```python
from build123d import *

# Parameters (mm, degrees)
SKETCH1_W           = 57
SKETCH1_H           = 100
BOSS_EXTRUDE1_DEPTH = 80
SKETCH3_W           = 75
SKETCH3_H           = 90
CUT_EXTRUDE1_DEPTH  = 52
SKETCH4_R           = 4.025
CUT_EXTRUDE2_DEPTH  = 114.213294272
BOSS_EXTRUDE2_DEPTH = 30
CUT_EXTRUDE5_REACH  = 112.223
SKETCH8_W           = 85
SKETCH8_H           = 40
SKETCH5_R           = 5
SKETCH5_R_2         = 1.5
CUT_EXTRUDE3_DEPTH  = 141.791512528
SKETCH9_R           = 11
SKETCH9_R_2         = 3
CUT_EXTRUDE6_DEPTH  = 47.5
FILLET1_R           = 1
FILLET2_R           = 5


with BuildPart() as part:
    # Sketch1 → Boss-Extrude1 (new body)
    with BuildSketch(Plane(origin=(0, 0, 0), x_dir=(1, 0, 0), z_dir=(0, 1, 0))):
        Rectangle(SKETCH1_W, SKETCH1_H)
    extrude(amount=BOSS_EXTRUDE1_DEPTH)

    # Sketch3 → Cut-Extrude1 (cut)
    with BuildSketch(Plane(origin=(28.5, 40, 0), x_dir=(0, 1, 0), z_dir=(-1, 0, 0))):
        with Locations((2.5, 0)):
            Rectangle(SKETCH3_W, SKETCH3_H)
    extrude(amount=CUT_EXTRUDE1_DEPTH, mode=Mode.SUBTRACT)

    # Sketch4 → Cut-Extrude2 (cut, through all)
    with BuildSketch(Plane(origin=(-40, 5, 0), x_dir=(-1, 0, 0), z_dir=(0, -1, 0))):
        with Locations(Location((-40, 0, 0), (0, 0, 90))):
            Circle(SKETCH4_R)
    extrude(amount=CUT_EXTRUDE2_DEPTH, mode=Mode.SUBTRACT)

    # Sketch7 → Boss-Extrude2 (add)
    with BuildSketch(Plane.ZY.offset(28.5)):
        Polygon((-50, 80), (-42.5, 80), (-42.5, 40), (42.5, 40), (42.5, 80), (50, 80), (50, 35), (-50, 35), align=None)
    extrude(amount=BOSS_EXTRUDE2_DEPTH)

    # Sketch8 → Cut-Extrude5 (cut, up to next)
    with BuildSketch(Plane.ZY.offset(28.5), mode=Mode.PRIVATE) as cut_extrude5_sk1:
        with Locations((0, 60)):
            Rectangle(SKETCH8_W, SKETCH8_H)
    cut_extrude5_tool1 = extrude(cut_extrude5_sk1.sketch, amount=-CUT_EXTRUDE5_REACH, mode=Mode.PRIVATE) & part.part
    add(cut_extrude5_tool1.solids().sort_by_distance((-28.5, 60, 0))[0], mode=Mode.SUBTRACT)

    # Sketch5 → Cut-Extrude3 (cut, through all)
    with BuildSketch(Plane(origin=(0, 0, -50), x_dir=(-1, 0, 0), z_dir=(0, 0, -1))):
        with Locations((44.5, 62.5)):
            Circle(SKETCH5_R)
        with Locations((-23.1, 58.1)):
            Circle(SKETCH5_R_2)
        with Locations((8.1, 58.1)):
            Circle(SKETCH5_R_2)
        with Locations((8.1, 26.9)):
            Circle(SKETCH5_R_2)
        with Locations((-23.1, 26.9)):
            Circle(SKETCH5_R_2)
        with Locations((10.5, 63.6)):
            Circle(SKETCH5_R_2)
        with Locations((18.5, 38.5)):
            Circle(SKETCH5_R_2)
        with BuildLine():
            Line((-1.5, 31), (-7.5, 31))
            ThreePointArc((-7.5, 31), (-19, 42.5), (-7.5, 54))
            Line((-7.5, 54), (-1.5, 54))
            ThreePointArc((-1.5, 54), (10, 42.5), (-1.5, 31))
        make_face()
    extrude(amount=-CUT_EXTRUDE3_DEPTH, mode=Mode.SUBTRACT)

    # Sketch9 → Cut-Extrude6 (cut, symmetric)
    with BuildSketch(Plane.XY):
        with Locations((-44.5, 62.5)):
            Circle(SKETCH9_R)
        with Locations((-10.5, 63.6)):
            Circle(SKETCH9_R_2)
        with Locations((-18.5, 38.5)):
            Circle(SKETCH9_R_2)
    extrude(amount=CUT_EXTRUDE6_DEPTH, both=True, mode=Mode.SUBTRACT)

    # Fillet1
    fillet1_edges = [part.edges().sort_by_distance(p)[0] for p in [
        (-23.5, 42.5, 45),
        (-23.5, 42.5, -45),
        (-23.5, 60, 42.5),
        (-23.5, 60, -42.5),
    ]]
    fillet(fillet1_edges, radius=FILLET1_R)

    # Fillet2
    fillet2_edges = [part.edges().sort_by_distance(p)[0] for p in [
        (-58.5, 80, 46.25),
        (-58.5, 80, -46.25),
    ]]
    fillet(fillet2_edges, radius=FILLET2_R)


solid = part.part
```
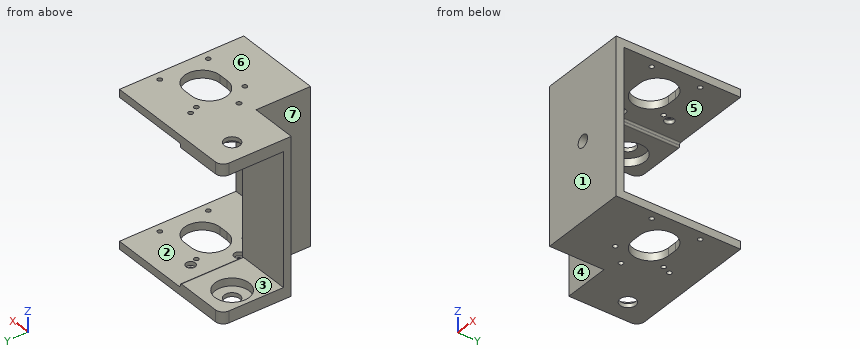
Verification items for the finished model (mm, model axes). Face numbers are marked on the shaded views. A direction names the side the tool comes from. Give positions to 0.01 mm unless a question says otherwise; leave off trailing zeros. Loops run counter-clockwise (first coordinate to the right, second up) from the corner with the lowest first, then second, coordinate; pieces in that order, holes last. Notation, with made-up numbers: M 30.25,46.25 L 53.25,46.25 A23 ccw 53.25,73.25 Z; hole C 68,4 d7. An arc over 180 degrees is marked long. Return JSON: item names as keys, results as strings.
1) Section check B-B, the plane z = -19. Enter the section's corners in (x, y), and give its area (3 significant figures).
Findings:
{"outline": "M -58.5,35 L -28.5,35 L -28.5,0 L 28.5,0 L 28.5,5 L -23.5,5 L -23.5,40 L -58.5,40 Z", "area": "610 mm2"}
2) Section check A-A, the plane y = 26.9. Enter the section's corners in (x, z).
Findings:
{"outline": "M -28.5,-50 L -9.6,-50 L -9.6,-45 L -22.5,-45 A1 cw -23.5,-44 L -23.5,44 A1 cw -22.5,45 L -9.6,45 L -9.6,50 L -28.5,50 Z; M -6.6,-50 L 21.6,-50 L 21.6,-45 L -6.6,-45 Z; M -6.6,45 L 21.6,45 L 21.6,50 L -6.6,50 Z; M 24.6,-50 L 28.5,-50 L 28.5,-45 L 24.6,-45 Z; M 24.6,45 L 28.5,45 L 28.5,50 L 24.6,50 Z"}
3) Material ranges on L1, parallel to Z at x = 20, y = 16.5; L2, parallel to Z at x = -47, y = 57.5; L3, parallel to X at y = 26, z = -47, recorded low to high. Write a range as [from, to].
Findings:
{"L1": "z = [-50, -45], [45, 50]", "L2": "z = [-50, -47.5], [47.5, 50]", "L3": "x = [-28.5, -9.3], [-6.9, 21.9], [24.3, 28.5]"}
4) Mould release check, pull along Z, two halves, no side actions. Record for the marked faces 5, 6 and 7: released by +Z, released by -Z, zero draft, split by the parting line, or undercut.
Findings:
{"face 5": "undercut", "face 6": "released by +Z", "face 7": "zero draft"}
5) Section check C-C, the plane x = -18.5. Enter the section's corners in (y, z), and give its area (4 significant figures).
Findings:
{"outline": "M 0,-50 L 37,-50 L 37,-47.5 L 35.5,-47.5 L 35.5,-45 L 5,-45 L 5,45 L 35.5,45 L 35.5,47.5 L 37,47.5 L 37,50 L 0,50 Z; M 40,-50 L 80,-50 L 80,-45 L 41.5,-45 L 41.5,-47.5 L 40,-47.5 Z; M 40,47.5 L 41.5,47.5 L 41.5,45 L 80,45 L 80,50 L 40,50 Z", "area": "1,205 mm2"}
6) Gauge pin test, flat ends, axial feed: P1, Ø12, axis at x = 9, z = -20, coming from the -Y side; P2, Ø3, axis at y = 43, z = -33.5, coming from the +X side; P3, Ø8, axis at x = -49.5, z = -38, coming from the -Y side; P4, Ø17.5, axis at y = 11, z = 22.5, coming from the -X side. Record the tip position at first contact, or that the pin passes through.
Findings:
{"P1": "stops at y = 0", "P2": "passes through", "P3": "stops at y = 35", "P4": "stops at x = -28.5"}
7) Section check D-D, the plane x = 0. Enter the section's corners in (y, z) (3 decimals), and give its area (3 significant figures).
Findings:
{"outline": "M 0,-50 L 31.098,-50 L 31.098,-45 L 5,-45 L 5,-4.025 L 0,-4.025 Z; M 0,4.025 L 5,4.025 L 5,45 L 31.098,45 L 31.098,50 L 0,50 Z; M 53.902,-50 L 80,-50 L 80,-45 L 53.902,-45 Z; M 53.902,45 L 80,45 L 80,50 L 53.902,50 Z", "area": "982 mm2"}
8) Tool access check on the marked faces 1, 2, 3 and 4. Record the directions out of +Z, -Z, +X, -X, +Y, -Y that give a thin tool (end or side, any length) a straight path to the whole face; none if there is none.
Findings:
{"face 1": "+Z, -Z, +X, -X, -Y", "face 2": "+X, +Y", "face 3": "+X, -X, +Y", "face 4": "+Z, -Z, -X, -Y"}
